Could you check a few things on this model? Use its own coordinates, in mm. A direction names the side the tool comes from. Coordinates: 2 decimals unless noted, no trailing zeros. Order: outer loops, then holes, each group sorted by start corner. A loop starts at its lowest first (then second) coordinate and runs counter-clockwise, first axis right, second up. Notation, with made-up numbers: (27.25, 12.25) -> (34.25, 12.25) arc R32 cw to (34.25, 45.25) -> close; hole circle Ø10 at (87, -31). An arc over 180 degrees is marked (long way). Put each result on its own line as item: value. Start each with the question number.
Q1. We'd pull the mould along Y, two halves only. Please class faces 5 (the face through (94.028, -394.734, 27.653)), 6 (the face through (92, -336, 13)), 7 (the face through (93, -409.5, 14)): +Y half, -Y half, draft (parallel to the pull), parting line (faces both ways), or undercut.
Q2. Will these pins go through, and if not, where does the flat tip stop? pin 1 (3.5 mm diameter, centred on y = -371.5, z = 29.5, fed in from -X); pin 2 (1.2 mm diameter, centred on x = 88.5, y = -399.5, fed in from -Z); pin 3 (1.5 mm diameter, centred on x = 88.5, y = -392.5, fed in from +Z); pin 4 (2.5 mm diameter, centred on y = -318.5, z = 30, fed in from -X).
Q3. If we section it at A-A (y = -299.5): Please give me the cut outline in (x, z).
Q4. Please list where these lines run through material, in increasing order: line 1 along Z through (x, y) = (95.1, -331.5); line 2 along Z through (x, y) = (94.75, -355); line 3 along X through (y, z) = (-291.5, 13).
Q5. For faces 1 (the face through (88.5, -315.6, 25.5)), 2 (the face through (94.028, -289.548, -2.066)), 3 (the face through (88.5, -315.4, 1.5)), 4 (the face through (88, -269, 27.5)), which set-ups out of +Z, -Z, +X, -X, +Y, -Y let a thin tool reach every point of the face, with its end or its side?
from build123d import *

# Parameters (mm, degrees)
PAD004_DEPTH    = 144
SKETCH051_W     = 40
SKETCH051_H     = 144
PAD005_DEPTH    = 4
SKETCH052_R     = 1.5
POCKET019_DEPTH = 5
SKETCH014_R     = 2
POCKET020_DEPTH = 4
SKETCH015_R     = 4
POCKET021_DEPTH = 7


with BuildPart() as leftback001:
    # Sketch050 → Pad004 (new body)
    with BuildSketch(Plane.XZ):
        Polygon((0, 0), (0, 10), (7, 10), (7, 14), (-4, 14), (-4, -14), (7, -14), (7, -10), (0, -10), align=None)
    extrude(amount=PAD004_DEPTH)

    # Sketch051 (on Face4 of Pad004) → Pad005 (join)
    with BuildSketch(Plane(origin=(-4, 0, 0), x_dir=(0, 0, -1), z_dir=(-1, 0, 0))):
        with Locations((0, 72)):
            Rectangle(SKETCH051_W, SKETCH051_H)
    extrude(amount=-PAD005_DEPTH)

    # Sketch052 (on Face14 of Pad005) → Pocket019 (cut)
    with BuildSketch(Plane(origin=(-4, 0, 0), x_dir=(0, 0, -1), z_dir=(-1, 0, 0))):
        with Locations((0, 74)):
            Circle(SKETCH052_R)
    extrude(amount=-POCKET019_DEPTH, mode=Mode.SUBTRACT)

    # Sketch014 (on Face13 of Pocket019) → Pocket020 (cut)
    with BuildSketch(Plane(origin=(-4, 0, 0), x_dir=(0, 0, -1), z_dir=(-1, 0, 0))):
        with Locations((-16, 10)):
            Circle(SKETCH014_R)
        with Locations((-16, 18)):
            Circle(SKETCH014_R)
        with Locations((-16, 26)):
            Circle(SKETCH014_R)
        with Locations((-16, 34)):
            Circle(SKETCH014_R)
        with Locations((-16, 42)):
            Circle(SKETCH014_R)
        with Locations((-16, 50)):
            Circle(SKETCH014_R)
        with Locations((-16, 58)):
            Circle(SKETCH014_R)
        with Locations((-16, 66)):
            Circle(SKETCH014_R)
        with Locations((-16, 138)):
            Circle(SKETCH014_R)
        with Locations((-16, 130)):
            Circle(SKETCH014_R)
        with Locations((-16, 122)):
            Circle(SKETCH014_R)
        with Locations((-16, 114)):
            Circle(SKETCH014_R)
        with Locations((-16, 106)):
            Circle(SKETCH014_R)
        with Locations((-16, 98)):
            Circle(SKETCH014_R)
        with Locations((-16, 90)):
            Circle(SKETCH014_R)
        with Locations((-16, 82)):
            Circle(SKETCH014_R)
        with Locations((-16, 74)):
            Circle(SKETCH014_R)
        with Locations((16, 138)):
            Circle(SKETCH014_R)
        with Locations((16, 130)):
            Circle(SKETCH014_R)
        with Locations((16, 122)):
            Circle(SKETCH014_R)
        with Locations((16, 114)):
            Circle(SKETCH014_R)
        with Locations((16, 106)):
            Circle(SKETCH014_R)
        with Locations((16, 98)):
            Circle(SKETCH014_R)
        with Locations((16, 90)):
            Circle(SKETCH014_R)
        with Locations((16, 82)):
            Circle(SKETCH014_R)
        with Locations((16, 74)):
            Circle(SKETCH014_R)
        with Locations((16, 66)):
            Circle(SKETCH014_R)
        with Locations((16, 58)):
            Circle(SKETCH014_R)
        with Locations((16, 50)):
            Circle(SKETCH014_R)
        with Locations((16, 42)):
            Circle(SKETCH014_R)
        with Locations((16, 34)):
            Circle(SKETCH014_R)
        with Locations((16, 26)):
            Circle(SKETCH014_R)
        with Locations((16, 18)):
            Circle(SKETCH014_R)
        with Locations((16, 10)):
            Circle(SKETCH014_R)
    extrude(amount=-POCKET020_DEPTH, mode=Mode.SUBTRACT)

    # Sketch015 (on Face15 of Pocket019) → Pocket021 (cut)
    with BuildSketch(Plane(origin=(0, 0, 0), x_dir=(0, 0, 1), z_dir=(1, 0, 0))):
        with Locations((-16, 10)):
            Circle(SKETCH015_R)
        with Locations((-16, 18)):
            Circle(SKETCH015_R)
        with Locations((-16, 26)):
            Circle(SKETCH015_R)
        with Locations((-16, 34)):
            Circle(SKETCH015_R)
        with Locations((-16, 42)):
            Circle(SKETCH015_R)
        with Locations((-16, 50)):
            Circle(SKETCH015_R)
        with Locations((-16, 58)):
            Circle(SKETCH015_R)
        with Locations((-16, 66)):
            Circle(SKETCH015_R)
        with Locations((-16, 138)):
            Circle(SKETCH015_R)
        with Locations((-16, 130)):
            Circle(SKETCH015_R)
        with Locations((-16, 122)):
            Circle(SKETCH015_R)
        with Locations((-16, 114)):
            Circle(SKETCH015_R)
        with Locations((-16, 106)):
            Circle(SKETCH015_R)
        with Locations((-16, 98)):
            Circle(SKETCH015_R)
        with Locations((-16, 90)):
            Circle(SKETCH015_R)
        with Locations((-16, 82)):
            Circle(SKETCH015_R)
        with Locations((-16, 74)):
            Circle(SKETCH015_R)
        with Locations((16, 138)):
            Circle(SKETCH015_R)
        with Locations((16, 130)):
            Circle(SKETCH015_R)
        with Locations((16, 122)):
            Circle(SKETCH015_R)
        with Locations((16, 114)):
            Circle(SKETCH015_R)
        with Locations((16, 106)):
            Circle(SKETCH015_R)
        with Locations((16, 98)):
            Circle(SKETCH015_R)
        with Locations((16, 90)):
            Circle(SKETCH015_R)
        with Locations((16, 82)):
            Circle(SKETCH015_R)
        with Locations((16, 74)):
            Circle(SKETCH015_R)
        with Locations((16, 66)):
            Circle(SKETCH015_R)
        with Locations((16, 58)):
            Circle(SKETCH015_R)
        with Locations((16, 50)):
            Circle(SKETCH015_R)
        with Locations((16, 42)):
            Circle(SKETCH015_R)
        with Locations((16, 34)):
            Circle(SKETCH015_R)
        with Locations((16, 26)):
            Circle(SKETCH015_R)
        with Locations((16, 18)):
            Circle(SKETCH015_R)
        with Locations((16, 10)):
            Circle(SKETCH015_R)
    extrude(amount=POCKET021_DEPTH, mode=Mode.SUBTRACT)


with BuildPart() as leftback001_1:
    # Body016 placement: moved
    add(leftback001.part.moved(Location((-92, -265.5, 13.5))))


with BuildPart() as rightback001:
    # Part__Mirroring004: instance of LeftBack001
    add(leftback001_1.part.mirror(Plane(origin=(0, 0, 0), x_dir=(0, -1, 0), z_dir=(1, 0, 0))))


solid = rightback001.part
The answers:
1. face 5: undercut
1. face 6: draft
1. face 7: -Y half
2. pin 1: through
2. pin 2: z = -0.5
2. pin 3: z = 27.5
2. pin 4: x = 92
3. outline: (85, 1.5) -> (92, 1.5) -> (92, -0.5) -> (96, -0.5) -> (96, 27.5) -> (92, 27.5) -> (92, 25.5) -> (85, 25.5) -> (85, 23.5) -> (92, 23.5) -> (92, 3.5) -> (85, 3.5) -> close; (92, -6.5) -> (96, -6.5) -> (96, -4.5) -> (92, -4.5) -> close; (92, 31.5) -> (96, 31.5) -> (96, 33.5) -> (92, 33.5) -> close
4. line 1: -6.5 to -4.5, -0.5 to 27.5, 31.5 to 33.5
4. line 2: -6.5 to -4.44, -0.56 to 27.56, 31.44 to 33.5
4. line 3: 92 to 96
5. face 1: +Z, -X
5. face 2: +X, -X
5. face 3: -Z, -X
5. face 4: +Z, -X, +Y, -Y
